from build123d import *

# Parameters (mm, degrees)
F1_DEPTH = 152.4


# Not quite as in the source:
# - ends of sketch curves that miss each other by under 0.0002 mm in the source are joined


with BuildPart() as f1:
    # F0 (on Front) → F1 (new body)
    with BuildSketch(Plane.XZ):
        with BuildLine():
            Line((-12.3838716, -0.0228854), (-12.3838716, -4.7218854))
            Line((-12.3838716, -4.7218854), (12.383897, -4.7218854))
            Line((12.383897, -4.7218854), (12.383897, -0.7239254))
            ThreePointArc((12.383897, -0.7239254), (9.9901302454, 1.6896267796), (7.1382289827, -0.1602538356))
            Line((7.1382289827, -0.1602538356), (6.1675772, 0.81153))
            ThreePointArc((6.1675772, 0.81153), (5.9240303947, 0.9642906727), (5.6377868977, 0.9375583076))
            ThreePointArc((5.6377868977, 0.9375583076), (0.7948702497, 0.8064034512), (-3.3428712434, 3.3263562022))
            ThreePointArc((-3.3428712434, 3.3263562022), (-7.7001712998, 4.4538085328), (-10.1053789302, 0.6495786484))
            ThreePointArc((-10.1053789302, 0.6495786484), (-11.4361565644, 0.9623164645), (-12.3838716, -0.0228854))
        make_face()
    extrude(amount=F1_DEPTH)


solid = f1.part
Verification items for the finished model (mm, model axes). Round coordinates to 2 decimals unless told otherwise and drop trailing zeros. Write each loop counter-clockwise with the first axis right and the second up, starting at its lowest first coordinate (ties: lowest second). Pieces come first, ordered by that corner, then holes.
(1) Section check A-A (y = -8.5). Enter the section's corners in (x, z), plus the area to 3 significant figures.
Returned:
outline: (-12.38, -4.72) - (12.38, -4.72) - (12.38, -0.72) arc R2.69 ccw to (7.14, -0.16) - (6.17, 0.81) arc R0.45 ccw to (5.64, 0.94) arc R8.56 cw to (-3.34, 3.33) arc R3.82 ccw to (-10.11, 0.65) arc R1.38 ccw to (-12.38, -0.02) - close
area: 164 mm2
(2) Mould release check, pull along X, two halves, no side actions. Record for faces 1 (the cylindrical face through (0.86, -75.13, 0.79)), 2 (the flat face through (0, 0, -1)), 3 (the cylindrical face through (10.041, -75.133, 1.684)), 4 (the flat face through (-12.384, -75, -2)): pulls with the +X half, pulls with the -X half, needs draft (parallel to the pull), parting line crosses it, or undercut.
Returned:
face 1: undercut
face 2: needs draft
face 3: undercut
face 4: pulls with the -X half
(3) Material ranges on line 1 (Z direction, x = 0.75, y = -26.5); line 2 (X direction, y = -118.5, z = 0.25); line 3 (Z direction, x = 7, y = -32.5), recorded low to high.
Returned:
line 1: z = -4.72 to 0.82
line 2: x = -12.28 to 6.73, 7.31 to 12.09
line 3: z = -4.72 to -0.02
(4) Depth check by flat-ended pin: pin 1 Ø3 at (x, y) = (-2.5, -26) entering from +Z; pin 2 Ø10 at (x, y) = (4, -56) entering from +Z; pin 3 Ø6 at (x, y) = (-8.5, -61.5) entering from +Z. Enter the tip coordinate at first touch or a pass-through.
Returned:
pin 1: stops at z = 3.96
pin 2: stops at z = 1.61
pin 3: stops at z = 4.72
(5) Section check C-C (x = -8.75). Enter the section's corners in (y, z), plus the area to 3 significant figures.
Returned:
outline: (-152.4, -4.72) - (0, -4.72) - (0, 3.83) - (-152.4, 3.83) - close
area: 1,300 mm2
(6) Section check B-B (x = 1.75). Enter the section's corners in (y, z), plus the area to 3 significant figures.
Returned:
outline: (-152.4, -4.72) - (0, -4.72) - (0, 0.61) - (-152.4, 0.61) - close
area: 813 mm2
